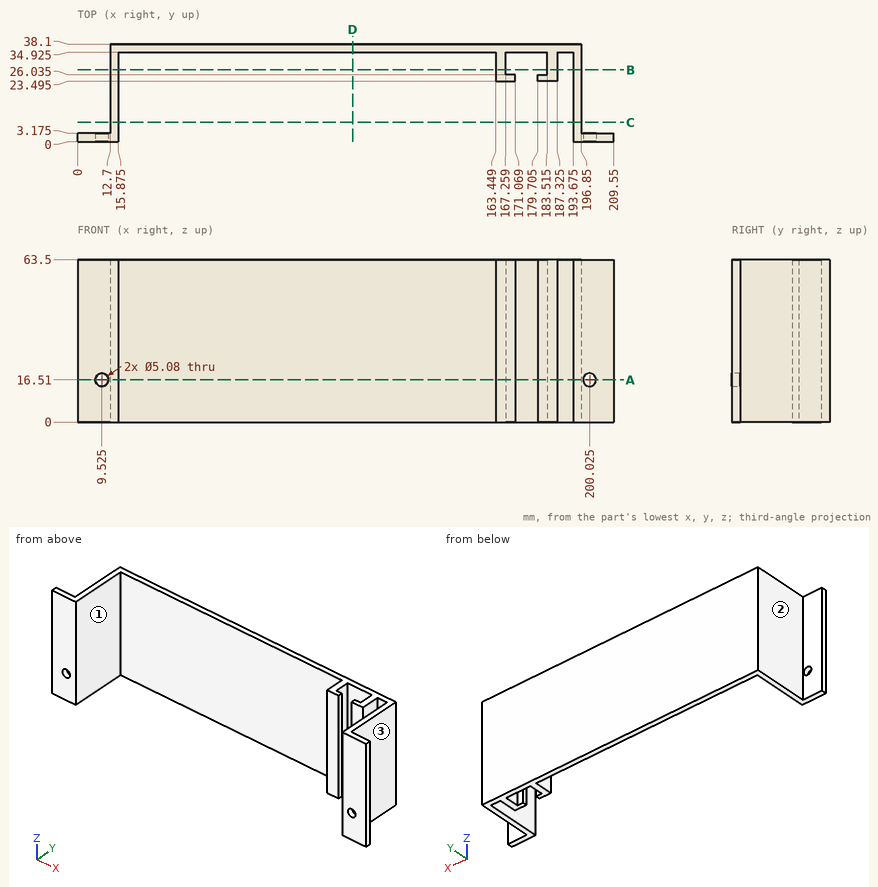
Drawing for the job (mm, zero at the part's lowest x, y, z). A direction names the side the tool comes from. Round coordinates to 2 decimals unless told otherwise and drop trailing zeros. Loops run counter-clockwise (first coordinate to the right, second up) from the corner with the lowest first, then second, coordinate; pieces in that order, holes last. Notation, with made-up numbers: (-35, 46.25) -> (-30, 46.25) arc R37 ccw to (-30, 83.25) -> close; hole circle Ø8 at (53.5, -26.75). An arc over 180 degrees is marked (long way). Answer in a Markdown table with one row per item.
Item 1: Drill centre lines: L1, parallel to X at y = 1.85, z = 16.51 (3 decimals); L2, parallel to X at y = 32.5, z = 8 (3 decimals); L3, parallel to X at y = 20, z = 59 (3 decimals). Where is each one in solid material? Low to high. Write a range as [from, to].
Answers below:
| item | result |
|---|---|
| L1 | x = [0, 6.985], [12.065, 15.875], [193.675, 197.485], [202.565, 209.55] |
| L2 | x = [12.7, 15.875], [163.449, 167.259], [183.515, 187.325], [193.675, 196.85] |
| L3 | x = [12.7, 15.875], [193.675, 196.85] |
Item 2: Saw through at D-D (x = 107.5). Write the cut outline in (y, z) (3 decimals), and give its area (3 significant figures).
Answers below:
| item | result |
|---|---|
| outline | (34.925, 0) -> (38.1, 0) -> (38.1, 63.5) -> (34.925, 63.5) -> close |
| area | 202 mm² |
Item 3: Saw through at C-C (y = 7.5). Write the cut outline in (x, z) (3 decimals).
Answers below:
| item | result |
|---|---|
| outline | (12.7, 0) -> (15.875, 0) -> (15.875, 63.5) -> (12.7, 63.5) -> close; (193.675, 0) -> (196.85, 0) -> (196.85, 63.5) -> (193.675, 63.5) -> close |
Item 4: Saw through at B-B (y = 28). Write the cut outline in (x, z) (3 decimals), and give its area (3 significant figures).
Answers below:
| item | result |
|---|---|
| outline | (12.7, 0) -> (15.875, 0) -> (15.875, 63.5) -> (12.7, 63.5) -> close; (163.449, 0) -> (167.259, 0) -> (167.259, 63.5) -> (163.449, 63.5) -> close; (183.515, 0) -> (187.325, 0) -> (187.325, 63.5) -> (183.515, 63.5) -> close; (193.675, 0) -> (196.85, 0) -> (196.85, 63.5) -> (193.675, 63.5) -> close |
| area | 887 mm² |
Item 5: Which spindle directions (+Z, -Z, +X, -X, +Y, -Y) get a long thin tool onto all of the face, cutting with end or side? Do the marked faces 1, 2 and 3. Say none if no direction does.
Answers below:
| item | result |
|---|---|
| face 1 | +Z, -Z, -Y |
| face 2 | +Z, -Z, -X, +Y |
| face 3 | +Z, -Z, +X, +Y |
Item 6: Saw through at A-A (z = 16.51). State how many separate pieces and enclosed holes the cut face has, and give its area (3 significant figures).
Answers below:
| item | result |
|---|---|
| separate pieces | 3 |
| enclosed holes | 0 |
| area | 961 mm² |
Item 7: Pin check, flat tips, straight feed: pin 1 (6 mm diameter, centred on x = 200.025, z = 16.51, fed in from +Y) (3 decimals); pin 2 (1.5 mm diameter, centred on x = 150, z = 50.5, fed in from -Y) (3 decimals); pin 3 (3 mm diameter, centred on y = 18, z = 37, fed in from +X). Stop position of each tip, or through.
Answers below:
| item | result |
|---|---|
| pin 1 | stops at y = 3.175 |
| pin 2 | stops at y = 34.925 |
| pin 3 | stops at x = 196.85 |
